Source: three-view drawing plus pictorial views. Frame: mm from the lowest corner of the part. Give positions to 0.01 mm unless a question says otherwise; leave off trailing zeros. Loops run counter-clockwise (first coordinate to the right, second up) from the corner with the lowest first, then second, coordinate; pieces in that order, holes last.
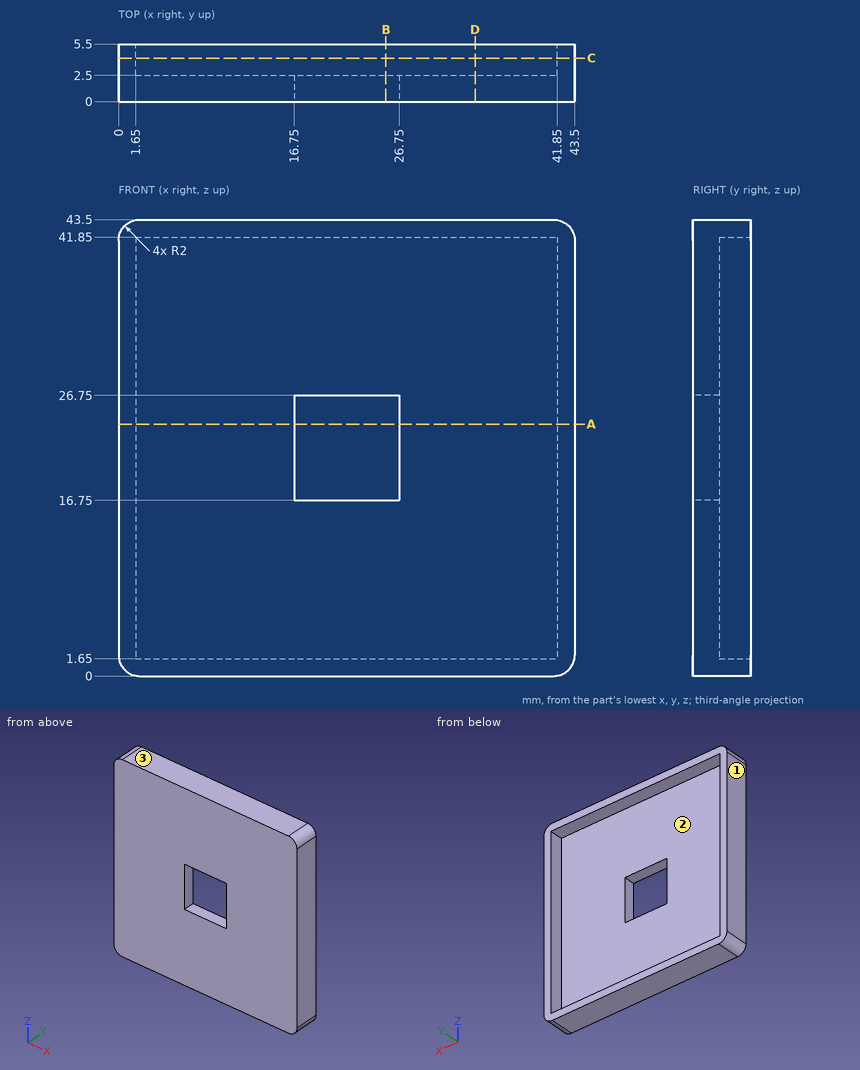
Q1. Section query C-C, the plane y = 4.15. Return loops of the section in (x, z).
Q2. Material intervals for probe 1 along Z at (x, y) = (26.5, 0.65); probe 2 along X at (y, z) = (3.85, 10.5), sorted ascending.
Q3. Section query A-A, the plane z = 24. Return loops of the section in (x, y).
Q4. Mould query, pull axis Z, two halves, no side actions, for the marked faces 1, 2 and 3. Classes: +Z half, -Z half, draft (parallel to the pull), parting line (faces both ways), or undercut.
Q5. Section query D-D, the plane x = 34. Return loops of the section in (y, z), and give its area (3 significant figures).
Q6. Pin query (flat end, axial travel): pin 1 Ø3 at (x, y) = (21.5, 1) entering from -Z; pin 2 Ø12 at (x, z) = (18, 15.5) entering from +Y. Return the tip coordinate at first contact, or that it passes through.
Q7. Section query B-B, the plane x = 25.5. Return loops of the section in (y, z).
Resolved:
1. outline: (0, 2) arc R2 ccw to (2, 0) - (41.5, 0) arc R2 ccw to (43.5, 2) - (43.5, 41.5) arc R2 ccw to (41.5, 43.5) - (2, 43.5) arc R2 ccw to (0, 41.5) - close; hole (1.65, 1.65) - (41.85, 1.65) - (41.85, 41.85) - (1.65, 41.85) - close
2. probe 1: z = 0 to 16.75, 26.75 to 43.5
2. probe 2: x = 0 to 1.65, 41.85 to 43.5
3. outline: (0, 0) - (16.75, 0) - (16.75, 2.5) - (1.65, 2.5) - (1.65, 5.5) - (0, 5.5) - close; (26.75, 0) - (43.5, 0) - (43.5, 5.5) - (41.85, 5.5) - (41.85, 2.5) - (26.75, 2.5) - close
4. face 1: draft
4. face 2: undercut
4. face 3: +Z half
5. outline: (0, 0) - (5.5, 0) - (5.5, 1.65) - (2.5, 1.65) - (2.5, 41.85) - (5.5, 41.85) - (5.5, 43.5) - (0, 43.5) - close
5. area: 119 mm2
6. pin 1: stops at z = 0
6. pin 2: stops at y = 2.5
7. outline: (0, 0) - (5.5, 0) - (5.5, 1.65) - (2.5, 1.65) - (2.5, 16.75) - (0, 16.75) - close; (0, 26.75) - (2.5, 26.75) - (2.5, 41.85) - (5.5, 41.85) - (5.5, 43.5) - (0, 43.5) - close
